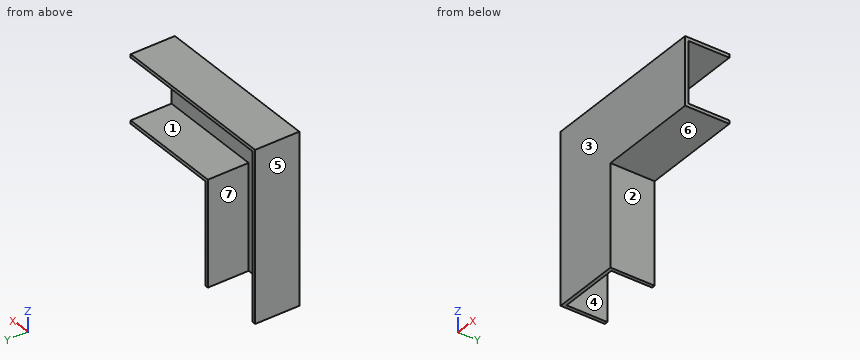
```python
from build123d import *

# Parameters (mm, degrees)
BOSS_EXTRUDE1_DEPTH = 330.2
CUT_EXTRUDE2_DEPTH  = 304.8


with BuildPart() as part:
    # Sketch1 → Boss-Extrude1 (new body)
    with BuildSketch(Plane(origin=(0, 0, 0), x_dir=(1, 0, 0), z_dir=(0, 1, 0))):
        Polygon((0, 0), (1270, 0), (1270, 508), (508, 508), (508, 1270), (0, 1270), align=None)
    extrude(amount=BOSS_EXTRUDE1_DEPTH)

    # Sketch2 → Cut-Extrude2 (cut)
    with BuildSketch(Plane(origin=(0, 330.2, 0), x_dir=(1, 0, 0), z_dir=(0, 1, 0))):
        Polygon((25.4, 1270), (25.4, 25.4), (1270, 25.4), (1270, 482.6), (482.6, 482.6), (482.6, 1270), align=None)
    extrude(amount=-CUT_EXTRUDE2_DEPTH, mode=Mode.SUBTRACT)


solid = part.part
```
Could you check a few things on this model? Use its own coordinates, in mm. Face numbers are marked on the shaded views. A direction names the side the tool comes from. Coordinates: 2 decimals unless noted, no trailing zeros. Write each loop counter-clockwise with the first axis right and the second up, starting at its lowest first coordinate (ties: lowest second). Pieces come first, ordered by that corner, then holes. Notation, with made-up numbers: (41.25, 0.25) -> (72.25, 0.25) arc R11 cw to (72.25, 16.25) -> close; hole circle Ø6 at (-3.75, 39). An arc over 180 degrees is marked (long way). One line per question, with ' | ' between items. Start each with the question number.
1. If we section it at D-D (x = 99.5): Please give me the cut outline in (y, z), and give its area (3 significant figures).
2. If we section it at C-C (z = -1055.5): Please give me the cut outline in (x, y).
3. For the marked faces 1, 2 and 3, which set-ups out of +Z, -Z, +X, -X, +Y, -Y let a thin tool reach every point of the face, with its end or its side?
4. If we section it at A-A (y = 242.5): Please give me the cut outline in (x, z).
5. If we section it at B-B (x = 553.5): Please give me the cut outline in (y, z), and give its area (3 significant figures).
6. Please list where these lines run through material, in increasing order: line 1 along X through (y, z) = (108, -723.5); line 2 along Z through (x, y) = (1168.5, 269); line 3 along Z through (x, y) = (93.5, 32).
7. Thinking about a two-plate mould opening in X: for the marked faces 4, 5, 6 and 7, which applies, pulls with the +X half, pulls with the -X half, needs draft (parallel to the pull), parting line crosses it, or undercut?
8. Will these pins go through, and if not, where does the flat tip stop? P1, Ø5, axis at y = 245, z = -588.5, coming from the +X side; P2, Ø3, axis at x = 992.5, y = 163.5, coming from the -Z side; P3, Ø12, axis at x = 293, z = -304.5, coming from the +Y side.
Return value:
1) outline: (0, -1270) -> (25.4, -1270) -> (25.4, -25.4) -> (330.2, -25.4) -> (330.2, 0) -> (0, 0) -> close | area: 40,000 mm²
2) outline: (0, 0) -> (508, 0) -> (508, 330.2) -> (482.6, 330.2) -> (482.6, 25.4) -> (25.4, 25.4) -> (25.4, 330.2) -> (0, 330.2) -> close
3) face 1: +X, +Y | face 2: -Z, +X, +Y, -Y | face 3: +Z, -Z, +X, -X, -Y
4) outline: (0, -1270) -> (25.4, -1270) -> (25.4, -25.4) -> (1270, -25.4) -> (1270, 0) -> (0, 0) -> close; (482.6, -1270) -> (508, -1270) -> (508, -508) -> (1270, -508) -> (1270, -482.6) -> (482.6, -482.6) -> close
5) outline: (0, -508) -> (330.2, -508) -> (330.2, -482.6) -> (25.4, -482.6) -> (25.4, -25.4) -> (330.2, -25.4) -> (330.2, 0) -> (0, 0) -> close | area: 28,400 mm²
6) line 1: x = 0 to 25.4, 482.6 to 508 | line 2: z = -508 to -482.6, -25.4 to 0 | line 3: z = -25.4 to 0
7) face 4: undercut | face 5: pulls with the -X half | face 6: needs draft | face 7: undercut
8) P1: stops at x = 508 | P2: stops at z = -508 | P3: stops at y = 25.4
